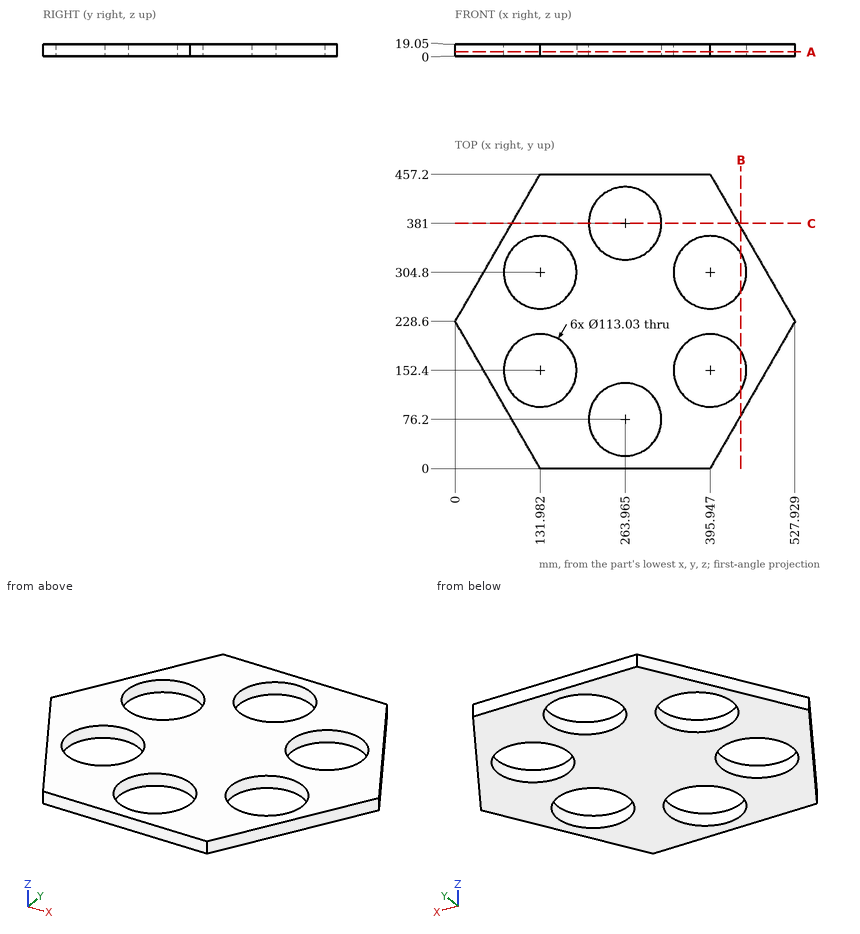
Study the drawing (mm; zero at the part's minimum x, y, z) and answer. Coordinates: 2 decimals unless noted, no trailing zeros. Loops run counter-clockwise (first coordinate to the right, second up) from the corner with the lowest first, then second, coordinate; pieces in that order, holes last. Notation, with made-up numbers: (76.25, 76.5) -> (110.25, 76.5) arc R13 cw to (110.25, 95.5) -> close; hole circle Ø8 at (59, 63). An arc over 180 degrees is marked (long way). Write each question's results on one line, items separated by ' | '. Start each with the question number.
1) Find section B-B on x = 444. Determine the outline of the cut face in (y, z), then the cut area to 3 significant figures.
2) Find section C-C on y = 381. Determine the outline of the cut face in (x, z), then the cut area to 3 significant figures.
3) Consider line 1 along X through (y, z) = (152.4, 9.75) (1 decimal); line 2 along X through (y, z) = (305.5, 14) (1 decimal); line 3 along Y through (x, z) = (139, 3.25). Determine where each line is inside the solid, lowest interval first.
4) Find section A-A on z = 6.75. Count the separate pieces of the cut face and the enclosed holes in it, then the cut area to 3 significant figures.
5) Flat-ended cylindrical pins translate along their axes: P1, Ø3, axis at y = 263.5, z = 10.5, coming from the -X side; P2, Ø10, axis at y = 276.5, z = 13, coming from the -X side; P3, Ø2, axis at y = 88.5, z = 13, coming from the -X side. Find the tip coordinate at first contact, or state that the pin passes through.
Response values:
1) outline: (83.23, 0) -> (122.65, 0) -> (122.65, 19.05) -> (83.23, 19.05) -> close; (182.15, 0) -> (275.05, 0) -> (275.05, 19.05) -> (182.15, 19.05) -> close; (334.55, 0) -> (373.97, 0) -> (373.97, 19.05) -> (334.55, 19.05) -> close | area: 3,270 mm^2
2) outline: (87.99, 0) -> (207.45, 0) -> (207.45, 19.05) -> (87.99, 19.05) -> close; (320.48, 0) -> (439.94, 0) -> (439.94, 19.05) -> (320.48, 19.05) -> close | area: 4,550 mm^2
3) line 1: x = 44 to 75.5, 188.5 to 339.4, 452.5 to 483.9 | line 2: x = 44.4 to 75.5, 188.5 to 339.4, 452.5 to 483.5 | line 3: y = 0 to 96.32, 208.48 to 248.72, 360.88 to 457.2
4) separate pieces: 1 | enclosed holes: 6 | area: 121,000 mm^2
5) P1: stops at x = 19.28 | P2: stops at x = 24.77 | P3: stops at x = 80.31
